```python
from build123d import *

# Parameters (mm, degrees)
EXTRUDE_1_DEPTH             = 50
HOLE_WIZARD_1_D             = 22
HOLE_WIZARD_1_DEPTH         = 100
HOLE_WIZARD_2_D             = 3.2
HOLE_WIZARD_2_DEPTH         = 100
HOLE_START                  = -3
HOLE_WIZARD_4_2_4_2_1_DEPTH = 3
RIB_1_REACH                 = 89.832
SKETCH_13_WALL_W            = 201.518173748
SKETCH_13_WALL_H            = 2.1
CHAMFER_1_SIZE              = 3


# Read off the part's stored shape, not the designer's step: Ø4.2 (4.2) 直径槽口1
with BuildPart() as part:
    # 草图1 → 凸台-拉伸1 (new body)
    with BuildSketch(Plane.XY):
        Polygon((0, 0), (50.5, 0), (50.5, 48.5), (53.5, 48.5), (53.5, -3), (0, -3), align=None)
    extrude(amount=EXTRUDE_1_DEPTH)

    # 孔1
    with Locations(Plane.ZY.offset(-50.5)):
        with Locations((25, 27.5)):
            Hole(HOLE_WIZARD_1_D / 2, depth=HOLE_WIZARD_1_DEPTH)

    # 孔2
    with Locations(Plane.ZY.offset(-50.5)):
        with Locations((10, 41.034802043), (41, 41.034802043), (41, 10.034802043), (10, 10.034802043)):
            Hole(HOLE_WIZARD_2_D / 2, depth=HOLE_WIZARD_2_DEPTH)

    # Ø4.2 (4.2) 直径槽口1 outline → Ø4.2 (4.2) 直径槽口1 (cut)
    with BuildSketch(Plane(origin=(0, 0, 0), x_dir=(1, 0, 0), z_dir=(0, 1, 0)).offset(HOLE_START)):
        with BuildLine():
            Line((11, -42.1), (41, -42.1))
            ThreePointArc((41, -42.1), (43.1, -40), (41, -37.9))
            Line((41, -37.9), (11, -37.9))
            ThreePointArc((11, -37.9), (8.9, -40), (11, -42.1))
        make_face()
        with BuildLine():
            Line((11, -12.1), (41, -12.1))
            ThreePointArc((41, -12.1), (43.1, -10), (41, -7.9))
            Line((41, -7.9), (11, -7.9))
            ThreePointArc((11, -7.9), (8.9, -10), (11, -12.1))
        make_face()
    extrude(amount=HOLE_WIZARD_4_2_4_2_1_DEPTH, mode=Mode.SUBTRACT)

    # 草图13 wall → 筋1 (add, up to next)
    with BuildSketch(Plane(origin=(44, 10, 50), x_dir=(-0.544988350595, -0.838443616301, 0), z_dir=(0.838443616301, -0.544988350595, 0)), mode=Mode.PRIVATE) as rib_1_sk1:
        with Locations((0, 1.05)):
            Rectangle(SKETCH_13_WALL_W, SKETCH_13_WALL_H)
    rib_1_tool1 = extrude(rib_1_sk1.sketch, amount=RIB_1_REACH, mode=Mode.PRIVATE) - part.part
    rib_1 = rib_1_tool1.solids().sort_by_distance((44, 10, 50))[0]
    add(rib_1)

    # 镜向1: 筋1 across plane
    add(rib_1.mirror(Plane.XY.offset(25)))

    # 倒角1
    chamfer_1_edges = [part.edges().sort_by_distance(p)[0] for p in [
        (52, 48.5, 50),
        (0, -1.5, 50),
        (52, 48.5, 0),
        (0, -1.5, 0),
    ]]
    chamfer(chamfer_1_edges, length=CHAMFER_1_SIZE)


solid = part.part
```
Part model, mm, in its own coordinate system. A direction names the side the tool comes from. Give positions to 0.01 mm unless a question says otherwise; leave off trailing zeros. Order: outer loops, then holes, each group sorted by start corner. A loop starts at its lowest first (then second) coordinate and runs counter-clockwise, first axis right, second up. Notation, with made-up numbers: (47, -27) - (65, -27) arc R21 cw to (65, 7) - close; hole circle Ø2 at (9, 60.5). An arc over 180 degrees is marked (long way). Use one line per item in the form item = value.
Item 1: Probe probe 1 along Y at (x, z) = (51.9, 41); probe 2 along Y at (x, z) = (51, 25); probe 3 along Z at (x, y) = (44.5, 1). List the from-to ranges inside material, lowest first. Write a range as from..to.
Solution:
probe_1 = -3..8.43, 11.63..39.43, 42.63..48.5
probe_2 = -3..16.5, 38.5..48.5
probe_3 = 0..2.1, 47.9..50
Item 2: Slice it at A-A on x = 36. Give the cut face in (y, z), and give its area (3 significant figures).
Solution:
outline = (-3, 0) - (0, 0) - (0, 7.9) - (-3, 7.9) - close; (-3, 12.1) - (0, 12.1) - (0, 37.9) - (-3, 37.9) - close; (-3, 42.1) - (0, 42.1) - (0, 50) - (-3, 50) - close
area = 125 mm2
Item 3: Slice it at B-B on z = 16.5. Give the cut face in (x, y), and give its area (3 significant figures).
Solution:
outline = (0, -3) - (53.5, -3) - (53.5, 20.52) - (50.5, 20.52) - (50.5, 0) - (0, 0) - close; (50.5, 34.48) - (53.5, 34.48) - (53.5, 48.5) - (50.5, 48.5) - close
area = 264 mm2
Item 4: Slice it at D-D on y = 19. Give the cut face in (x, z), and give its area (3 significant figures).
Solution:
outline = (49.85, 0) - (53.5, 0) - (53.5, 18.02) - (50.5, 18.02) - (50.5, 2.1) - (49.85, 2.1) - close; (49.85, 47.9) - (50.5, 47.9) - (50.5, 31.98) - (53.5, 31.98) - (53.5, 50) - (49.85, 50) - close
area = 111 mm2
Item 5: Pin check, flat tips, straight feed: pin 1 Ø14.5 at (x, y) = (41, 15) entering from -Z; pin 2 Ø6 at (x, z) = (11.5, 23) entering from +Y; pin 3 Ø3.5 at (y, z) = (41.03, 41) entering from -X. Stop position of each tip, or through.
Solution:
pin_1 = 0
pin_2 = 0
pin_3 = 50.5
Item 6: Slice it at C-C on y = 1. Give the cut face in (x, z).
Solution:
outline = (38.15, 0) - (53.5, 0) - (53.5, 50) - (38.15, 50) - (38.15, 47.9) - (50.5, 47.9) - (50.5, 2.1) - (38.15, 2.1) - close
Item 7: Two-plate mould, pull along X, no slides. Class faces 1 (the face through (26, -2, 37.9)), 2 (the face through (50.5, 13, 25)), 3 (the face through (52.021, 11.116, 11.179)): released by +X, released by -X, zero draft, split by the parting line, or undercut.
Solution:
face_1 = undercut
face_2 = released by -X
face_3 = zero draft
Item 8: Which spindle directions (+Z, -Z, +X, -X, +Y, -Y) get a long thin tool onto all of the face, cutting with end or side? Do faces 4 (the face through (53.5, 17, 19)), 5 (the face through (26, -2, 7.9)), 6 (the face through (25, 0, 25)). Say none if no direction does.
Solution:
face_4 = +Z, -Z, +X, +Y, -Y
face_5 = +Y, -Y
face_6 = -X, +Y
